```python
from build123d import *

# Parameters (mm, degrees)
SKETCH2_W           = 28
SKETCH2_H           = 35.2
SKETCH2_R           = 11
BOSS_EXTRUDE3_DEPTH = 7
SKETCH3_W           = 10
SKETCH3_H           = 3
BOSS_EXTRUDE4_DEPTH = 28
BOSS_EXTRUDE5_DEPTH = 3
BOSS_EXTRUDE6_START = -28
BOSS_EXTRUDE6_DEPTH = 3
SKETCH4_R           = 2
CUT_EXTRUDE1_DEPTH  = 101.089134132
BOSS_EXTRUDE7_START = 1
SKETCH2_3_W         = 28
SKETCH2_3_H         = 35.2
SKETCH2_3_R         = 11
SKETCH2_3_R_2       = 10.7
SKETCH2_3_R_3       = 9.65
SKETCH2_3_R_4       = 4.25
BOSS_EXTRUDE7_DEPTH = 1


with BuildPart() as part:
    # Sketch2 → Boss-Extrude3 (new body)
    with BuildSketch(Plane.XY.offset(-2.538447986)):
        with Locations((-78.732107824, 19.43595021)):
            Rectangle(SKETCH2_W, SKETCH2_H)
        with Locations((-78.732107824, 23.03595021)):
            Circle(SKETCH2_R, mode=Mode.SUBTRACT)
    extrude(amount=-BOSS_EXTRUDE3_DEPTH)

    # Sketch3 → Boss-Extrude4 (add)
    with BuildSketch(Plane.ZY.offset(92.732107824)):
        with Locations((-14.538447986, 3.33595021)):
            Rectangle(SKETCH3_W, SKETCH3_H)
    extrude(amount=-BOSS_EXTRUDE4_DEPTH)

    # Sketch3<3> → Boss-Extrude5 (add)
    with BuildSketch(Plane.ZY.offset(92.732107824)):
        Polygon((-19.538447986, 4.83595021), (-9.538447986, 4.83595021), (-9.538447986, 24.83595021), align=None)
    extrude(amount=-BOSS_EXTRUDE5_DEPTH)

    # Sketch3<4> → Boss-Extrude6 (add)
    with BuildSketch(Plane.ZY.offset(92.732107824).offset(BOSS_EXTRUDE6_START)):
        Polygon((-19.538447986, 4.83595021), (-9.538447986, 4.83595021), (-9.538447986, 24.83595021), align=None)
    extrude(amount=BOSS_EXTRUDE6_DEPTH)

    # Sketch4 → Cut-Extrude1 (cut, through all)
    with BuildSketch(Plane(origin=(0, 4.83595021, 0), x_dir=(1, 0, 0), z_dir=(0, 1, 0))):
        with Locations(Location((-72.732107824, 14.538447986, 0), (0, 0, 270))):
            Circle(SKETCH4_R)
        with Locations(Location((-84.732107824, 14.538447986, 0), (0, 0, 90))):
            Circle(SKETCH4_R)
    extrude(amount=-CUT_EXTRUDE1_DEPTH, mode=Mode.SUBTRACT)

    # Sketch2<3> → Boss-Extrude7 (add)
    # profile 1 of 4: a face of its own
    with BuildSketch(Plane.XY.offset(-2.538447986).offset(BOSS_EXTRUDE7_START)):
        with Locations((-78.732107824, 19.43595021)):
            Rectangle(SKETCH2_3_W, SKETCH2_3_H)
        with Locations((-78.732107824, 23.03595021)):
            Circle(SKETCH2_3_R, mode=Mode.SUBTRACT)
    # profile 2 of 4: a face of its own
    with BuildSketch(Plane.XY.offset(-2.538447986).offset(BOSS_EXTRUDE7_START)):
        with Locations((-78.732107824, 23.03595021)):
            Circle(SKETCH2_3_R)
        with Locations((-78.732107824, 23.03595021)):
            Circle(SKETCH2_3_R_2, mode=Mode.SUBTRACT)
    # profile 3 of 4: a face of its own
    with BuildSketch(Plane.XY.offset(-2.538447986).offset(BOSS_EXTRUDE7_START)):
        with Locations((-78.732107824, 23.03595021)):
            Circle(SKETCH2_3_R_2)
        with Locations((-78.732107824, 23.03595021)):
            Circle(SKETCH2_3_R_3, mode=Mode.SUBTRACT)
    # profile 4 of 4: a face of its own
    with BuildSketch(Plane.XY.offset(-2.538447986).offset(BOSS_EXTRUDE7_START)):
        with Locations((-78.732107824, 23.03595021)):
            Circle(SKETCH2_3_R_3)
        with Locations((-78.732107824, 23.03595021)):
            Circle(SKETCH2_3_R_4, mode=Mode.SUBTRACT)
    extrude(amount=-BOSS_EXTRUDE7_DEPTH)


solid = part.part
```
For this review, take the finished solid that the model builds, in its own axes (mm). A direction names the side the tool comes from. Round coordinates to 2 decimals unless told otherwise and drop trailing zeros. Write each loop counter-clockwise with the first axis right and the second up, starting at its lowest first coordinate (ties: lowest second). Pieces come first, ordered by that corner, then holes. Notation, with made-up numbers: (33.25, 45) -> (44.25, 45) arc R11 cw to (44.25, 49) -> close; hole circle Ø8 at (5.5, 28). An arc over 180 degrees is marked (long way). Use one line per item in the form item = value.
1) Take a section at C-C, the plane x = -75.5. Write out the cut boundary in (y, z).
Found:
outline = (1.84, -19.54) -> (4.84, -19.54) -> (4.84, -9.54) -> (12.52, -9.54) -> (12.52, -2.54) -> (20.28, -2.54) -> (20.28, -1.54) -> (1.84, -1.54) -> close; (25.8, -2.54) -> (33.55, -2.54) -> (33.55, -9.54) -> (37.04, -9.54) -> (37.04, -1.54) -> (25.8, -1.54) -> close
2) Mouldability with a two-part tool opening along X and no side actions: class faces 4 (the cylindrical face through (-71.05, 3.36, -13.46)), 5 (the flat face through (-92.732, 15, -8)), 6 (the flat face through (-79, 37.036, -5)) as +X half, -X half, draft (parallel to the pull), parting line (faces both ways), or undercut.
Found:
face_4 = undercut
face_5 = -X half
face_6 = draft
3) Tool access review of faces 1 (the flat face through (-67.732, 11, -12)), 2 (the cylindrical face through (-82.98, 23.22, -2.03)), 3 (the flat face through (-79, 18, -2.538)): name each direction out of +Z, -Z, +X, -X, +Y, -Y from which nothing blocks a thin tool from reaching the whole face with its end or side.
Found:
face_1 = -Z, +Y
face_2 = +Z, -Z
face_3 = -Z
4) Take a section at D-D, the plane z = -13.25. Write out the cut boundary in (x, y).
Found:
outline = (-92.73, 1.84) -> (-86.26, 1.84) -> (-86.26, 4.84) -> (-89.73, 4.84) -> (-89.73, 17.41) -> (-92.73, 17.41) -> close; (-83.2, 1.84) -> (-74.26, 1.84) -> (-74.26, 4.84) -> (-83.2, 4.84) -> close; (-71.2, 1.84) -> (-64.73, 1.84) -> (-64.73, 17.41) -> (-67.73, 17.41) -> (-67.73, 4.84) -> (-71.2, 4.84) -> close
5) To check wall thickness, follow L1, parallel to X at y = 10.5, z = -12.5; L2, parallel to Z at x = -83.75, y = 6.5; L3, parallel to Z at x = -84.5, y = 30.5. State the ranges of each line that lie inside material, in increasing order. Write a range as from..to.
Found:
L1 = -92.73..-89.73, -67.73..-64.73
L2 = -9.54..-1.54
L3 = -2.54..-1.54
6) Take a section at B-B, the plane y = 24. Write out the cut boundary in (x, z).
Found:
outline = (-92.73, -9.96) -> (-89.73, -9.96) -> (-89.73, -9.54) -> (-89.69, -9.54) -> (-89.69, -2.54) -> (-82.87, -2.54) -> (-82.87, -1.54) -> (-92.73, -1.54) -> close; (-74.59, -2.54) -> (-67.77, -2.54) -> (-67.77, -9.54) -> (-67.73, -9.54) -> (-67.73, -9.96) -> (-64.73, -9.96) -> (-64.73, -1.54) -> (-74.59, -1.54) -> close
7) Take a section at A-A, the plane z = -7.75. Write out the cut boundary in (x, y), and give its area (3 significant figures).
Found:
outline = (-92.73, 1.84) -> (-64.73, 1.84) -> (-64.73, 37.04) -> (-92.73, 37.04) -> close; hole circle Ø22 at (-78.73, 23.04)
area = 605 mm2
8) Clearance check with flat-ended pins moving along their axes: pin 1 (5 mm diameter, centred on x = -74.5, y = 16, fed in from -Z); pin 2 (12 mm diameter, centred on x = -89.5, y = 14, fed in from -Z); pin 3 (11 mm diameter, centred on x = -74.5, y = 27.5, fed in from -Z); pin 4 (7.5 mm diameter, centred on x = -78.73, y = 23.04, fed in from -Z). State where each tip first meets the part, or that it passes through.
Found:
pin_1 = -2.54
pin_2 = -17.95
pin_3 = -9.54
pin_4 = through
